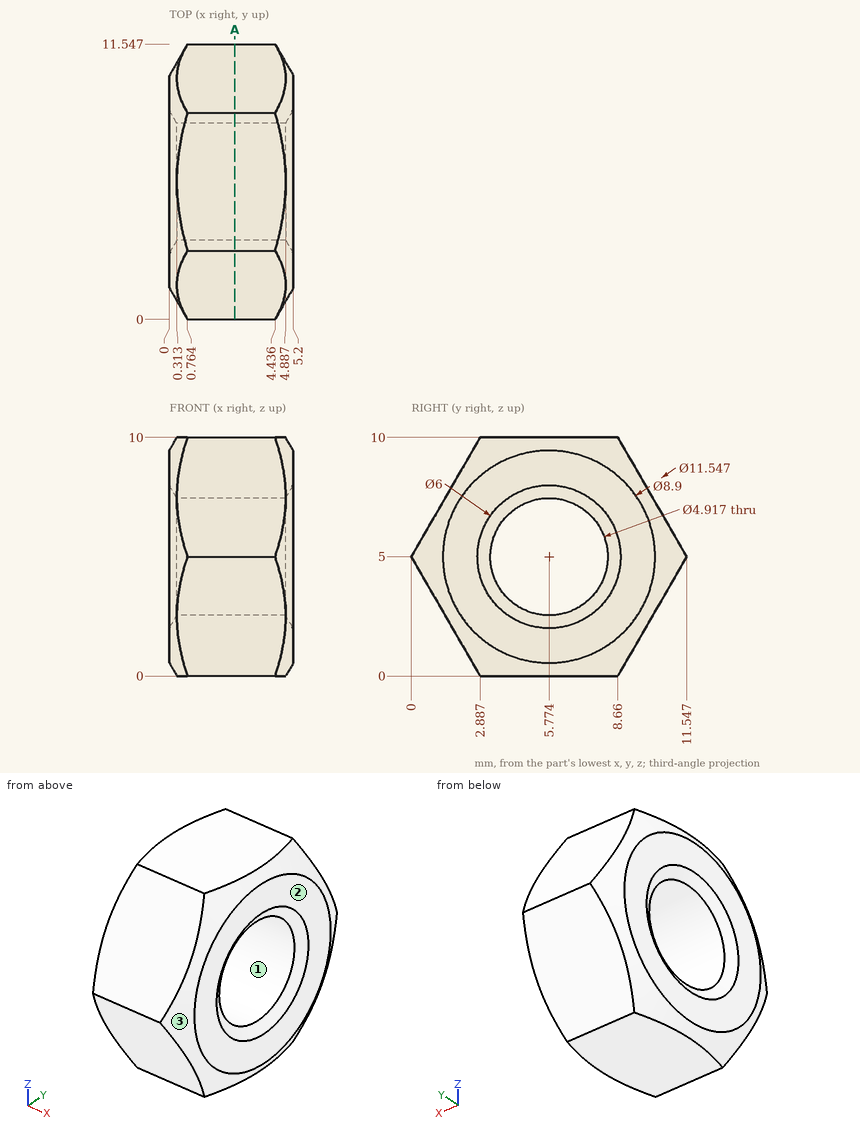
The drawing under review shows one solid part. Ordinate dimensions are in mm from its lowest x, y, z. Coordinates: 2 decimals unless noted, no trailing zeros. Order: outer loops, then holes, each group sorted by start corner. A loop starts at its lowest first (then second) coordinate and runs counter-clockwise, first axis right, second up. Notation, with made-up numbers: M 47.5,38 L 93.5,38 A19 ccw 93.5,55 Z; hole C 76,17.25 d9. An arc over 180 degrees is marked long. Use a Markdown table: item, result.
(1) Draft analysis for pull direction Z (two halves, no side actions). For the marked faces 1, 2 and 3, state which applies: released by +Z, released by -Z, zero draft, split by the parting line, or undercut.
Worked answers:
| item | result |
|---|---|
| face 1 | undercut |
| face 2 | zero draft |
| face 3 | split by the parting line |
(2) Wall thickness on probe 1 along Z at (x, y) = (2.7, 5.75); probe 2 along Z at (x, y) = (4.65, 6.25); probe 3 along Y at (x, z) = (3.5, 3.5) (1 decimal): over which ranges is each line inside the solid? List them lowest first.
Worked answers:
| item | result |
|---|---|
| probe 1 | z = 0 to 2.54, 7.46 to 10 |
| probe 2 | z = 0 to 2.59, 7.41 to 10 |
| probe 3 | y = 0.9 to 3.8, 7.7 to 10.7 |
(3) Add section A-A (x = 2.75). Give the boundary of the cut face in (y, z).
Worked answers:
| item | result |
|---|---|
| outline | M 0,5 L 2.89,0 L 8.66,0 L 11.55,5 L 8.66,10 L 2.89,10 Z; hole C 5.77,5 d4.92 |
(4) For P1, Ø3, axis at x = 4, y = 6.5, coming from the -Z side; P2, Ø4, axis at y = 5.77, z = 5, coming from the +X side, all flat-tipped, find the tip position at first contact; note any pin that passes through.
Worked answers:
| item | result |
|---|---|
| P1 | stops at z = 0 |
| P2 | passes through |
